from build123d import *

# Parameters (mm, degrees)
SKETCH1_R           = 38.1
SKETCH1_R_2         = 35.1
EXTRUDE_THIN1_DEPTH = 5
BOSS_EXTRUDE1_START = -10
BOSS_EXTRUDE1_DEPTH = 10
SKETCH3_R           = 2.375
CUT_EXTRUDE1_DEPTH  = 10
CIRPATTERN1_COUNT   = 4
SKETCH4_W           = 11
SKETCH4_H           = 10
BOSS_EXTRUDE2_DEPTH = 3
SKETCH5_R           = 2.1
CUT_EXTRUDE2_DEPTH  = 3
CIRPATTERN2_COUNT   = 4
CHAMFER1_SIZE       = 2.178281406
CHAMFER1_SIZE_2     = 2
SKETCH6_R           = 12
BOSS_EXTRUDE3_DEPTH = 5


with BuildPart() as part:
    # Sketch1 → Extrude-Thin1 (new, symmetric)
    with BuildSketch(Plane(origin=(0, 0, 0), x_dir=(1, 0, 0), z_dir=(0, 1, 0))):
        Circle(SKETCH1_R)
        Circle(SKETCH1_R_2, mode=Mode.SUBTRACT)
    extrude(amount=EXTRUDE_THIN1_DEPTH, both=True)

    # Sketch2 → Boss-Extrude1 (add)
    with BuildSketch(Plane(origin=(0, 5, 0), x_dir=(1, 0, 0), z_dir=(0, 1, 0)).offset(BOSS_EXTRUDE1_START)):
        with BuildLine():
            Line((-27.1, 6), (-27.1, -6))
            Line((-27.1, -6), (-33.700938133, -9.811053408))
            ThreePointArc((-33.700938133, -9.811053408), (-35.1, 0), (-33.700938133, 9.811053408))
            Line((-33.700938133, 9.811053408), (-27.1, 6))
        make_face()
    boss_extrude1 = extrude(amount=BOSS_EXTRUDE1_DEPTH)

    # Sketch3 → Cut-Extrude1 (cut)
    with BuildSketch(Plane(origin=(0, 5, 0), x_dir=(1, 0, 0), z_dir=(0, 1, 0))):
        with Locations(Location((-32, 0, 0), (0, 0, 270))):
            Circle(SKETCH3_R)
    cut_extrude1 = extrude(amount=-CUT_EXTRUDE1_DEPTH, mode=Mode.SUBTRACT)

    # CirPattern1: Boss-Extrude1, Cut-Extrude1 ×4 about axis
    cirpattern1_axis = Axis((0, 0, 0), (0, 1, 0))
    add([boss_extrude1.rotate(cirpattern1_axis, i * 360 / CIRPATTERN1_COUNT) for i in range(1, CIRPATTERN1_COUNT)])
    add([cut_extrude1.rotate(cirpattern1_axis, i * 360 / CIRPATTERN1_COUNT) for i in range(1, CIRPATTERN1_COUNT)], mode=Mode.SUBTRACT)

    # Sketch4 → Boss-Extrude2 (add)
    with BuildSketch(Plane.XY):
        with Locations((-42.6, 0)):
            Rectangle(SKETCH4_W, SKETCH4_H)
    boss_extrude2 = extrude(amount=BOSS_EXTRUDE2_DEPTH)

    # Sketch5 → Cut-Extrude2 (cut)
    with BuildSketch(Plane(origin=(0, 0, 0), x_dir=(-1, 0, 0), z_dir=(0, 0, -1))):
        with Locations((43.1, 0)):
            Circle(SKETCH5_R)
    cut_extrude2 = extrude(amount=-CUT_EXTRUDE2_DEPTH, mode=Mode.SUBTRACT)

    # CirPattern2: Boss-Extrude2, Cut-Extrude2 ×4 about axis
    cirpattern2_axis = Axis((0, 0, 0), (0, 1, 0))
    add([boss_extrude2.rotate(cirpattern2_axis, i * 360 / CIRPATTERN2_COUNT) for i in range(1, CIRPATTERN2_COUNT)])
    add([cut_extrude2.rotate(cirpattern2_axis, i * 360 / CIRPATTERN2_COUNT) for i in range(1, CIRPATTERN2_COUNT)], mode=Mode.SUBTRACT)

    # Chamfer1
    # the kernel refuses this chamfer: 2.178281406, 2 mm, written as the material it adds along each edge
    with BuildSketch(Plane(origin=(-3, -5, -37.981706123), x_dir=(-0.9944073694019739, 0, 0.10561242199214178), z_dir=(0, 1, 0))) as chamfer1_piece_1:
        with BuildLine():
            Line((2.056235734, 0), (-CHAMFER1_SIZE * 0.105612421996, -CHAMFER1_SIZE * 0.994407369435))
            Line((-CHAMFER1_SIZE * 0.105612421996, -CHAMFER1_SIZE * 0.994407369435), (0, 0))
            ThreePointArc((0, 0), (1.059779898, -0.013861107), (2.056235734, 0))
        make_face()
    extrude(amount=10)
    with BuildSketch(Plane(origin=(37.981706123, -5, -3), x_dir=(1, 0, 0), z_dir=(0, 1, 0)), Plane(origin=(3, -5, 37.981706123), x_dir=(0, 0, 1), z_dir=(0, 1, 0))) as chamfer1_piece_2:
        with BuildLine():
            Line((CHAMFER1_SIZE, 0), (-0.217164036, 2.044735967))
            ThreePointArc((-0.217164036, 2.044735967), (-0.098142335, 1.055316846), (0, 0))
            Line((0, 0), (CHAMFER1_SIZE, 0))
        make_face()
    extrude(amount=10)
    with BuildSketch(Plane(origin=(-38.1, -5, 0), x_dir=(0.026984720913872013, 0, -0.9996358461145741), z_dir=(0, 1, 0))) as chamfer1_piece_3:
        with BuildLine():
            Line((2.056235734, 0), (-CHAMFER1_SIZE_2 * 0.0269847209139, CHAMFER1_SIZE_2 * 0.999635846115))
            Line((-CHAMFER1_SIZE_2 * 0.0269847209139, CHAMFER1_SIZE_2 * 0.999635846115), (0, 0))
            ThreePointArc((0, 0), (1.057186648, 0.013863174), (2.056235734, 0))
        make_face()
    extrude(amount=10)

    # Sketch6 → Boss-Extrude3 (add, symmetric)
    with BuildSketch(Plane(origin=(0, 0, 0), x_dir=(1, 0, 0), z_dir=(0, 1, 0))):
        with BuildLine():
            Line((-2, 27.1), (-2, 14.866068747))
            ThreePointArc((-2, 14.866068747), (-10.606601718, 10.606601718), (-14.866068747, 2))
            Line((-14.866068747, 2), (-27.1, 2))
            Line((-27.1, 2), (-27.1, -2))
            Line((-27.1, -2), (-14.866068747, -2))
            ThreePointArc((-14.866068747, -2), (-10.606601718, -10.606601718), (-2, -14.866068747))
            Line((-2, -14.866068747), (-2, -27.1))
            Line((-2, -27.1), (2, -27.1))
            Line((2, -27.1), (2, -14.866068747))
            ThreePointArc((2, -14.866068747), (10.606601718, -10.606601718), (14.866068747, -2))
            Line((14.866068747, -2), (27.1, -2))
            Line((27.1, -2), (27.1, 2))
            Line((27.1, 2), (14.866068747, 2))
            ThreePointArc((14.866068747, 2), (10.606601718, 10.606601718), (2, 14.866068747))
            Line((2, 14.866068747), (2, 27.1))
            Line((2, 27.1), (-2, 27.1))
        make_face()
        with Locations(Location((0, 0, 0), (0, 0, 270))):
            Circle(SKETCH6_R, mode=Mode.SUBTRACT)
    extrude(amount=BOSS_EXTRUDE3_DEPTH, both=True)


solid = part.part
Design review of the part built by this model. Coordinates are the model's own, in mm. A direction names the side the tool comes from. Round coordinates to 2 decimals unless told otherwise and drop trailing zeros. Write each loop counter-clockwise with the first axis right and the second up, starting at its lowest first coordinate (ties: lowest second). Pieces come first, ordered by that corner, then holes. Notation, with made-up numbers: (32.25, -30) - (56.25, -30) arc R34 ccw to (56.25, 8) - close; hole circle Ø4 at (76.25, 61). An arc over 180 degrees is marked (long way). Use a Markdown table: item, result. Add a question column.
1. For faces 1 (the face through (-3, 1.2, -45.1)), 2 (the face through (45.4, 0.1, 0)), 3 (the face through (7.932, -0.07, -30.447)), list the 3-axis set-ups (+Z, -Z, +X, -X, +Y, -Y) from which the entire face can be reached by the end or side of a thin tool; tool diameter is ignored.
2. We need section A-A (z = 43.1). State the section outline as (x, y) points.
3. We need section B-B (y = 0). Count the separate pieces of the cut face and the enclosed holes in it, then the cut area to 3 significant figures.
4. We need section C-C (x = 7.5). State the section outline as (y, z) points, then the cut area to 3 significant figures.
5. Mouldability with a two-part tool opening along X and no side actions: class faces 4 (the face through (3, 1.2, 45.1)), 5 (the face through (-39.1, -0.1, -1)), 6 (the face through (27.1, 0, 4)) as +X half, -X half, draft (parallel to the pull), parting line (faces both ways), or undercut.
6. Wall thickness on probe 1 along Z at (x, y) = (-21.5, 3); probe 2 along X at (y, z) = (-3.75, -18): over which ranges is each line inside the solid? List them lowest first.
7. We need section D-D (z = -23.5). State the section outline as (x, y) points.
8. Clearance check with flat-ended pins moving along their axes: pin 1 (10 mm diameter, centred on x = 4, z = -8.5, fed in from +Y); pin 2 (4.5 mm diameter, centred on x = 3, y = -2.5, fed in from -Z); pin 3 (5.5 mm diameter, centred on x = -43.1, y = 0, fed in from -Z); pin 4 (1.2 mm diameter, centred on y = -2.5, z = -4, fed in from +X). State where each tip first meets the part, or that it passes through.
Output:
| question | item | result |
|---|---|---|
| 1 | face 1 | -Z, -X, +Y, -Y |
| 1 | face 2 | +Z, +X, +Y, -Y |
| 1 | face 3 | +Y, -Y |
| 2 | outline | (0, -5) - (3, -5) - (3, -2.1) - (0, -2.1) - close; (0, 2.1) - (3, 2.1) - (3, 5) - (0, 5) - close |
| 3 | separate pieces | 5 |
| 3 | enclosed holes | 9 |
| 3 | area | 1,640 mm2 |
| 4 | outline | (-5, -37.35) - (5, -37.35) - (5, -29.7) - (-5, -29.7) - close; (-5, -12.99) - (5, -12.99) - (5, -9.37) - (-5, -9.37) - close; (-5, 9.37) - (5, 9.37) - (5, 12.99) - (-5, 12.99) - close; (-5, 29.7) - (5, 29.7) - (5, 37.35) - (-5, 37.35) - close |
| 4 | area | 226 mm2 |
| 5 | face 4 | +X half |
| 5 | face 5 | -X half |
| 5 | face 6 | undercut |
| 6 | probe 1 | z = -31.45 to -27.74, -2 to 2, 27.74 to 31.45 |
| 6 | probe 2 | x = -33.58 to -30.13, -2 to 2, 30.13 to 33.58 |
| 7 | outline | (-29.99, -5) - (-26.07, -5) - (-26.07, 5) - (-29.99, 5) - close; (-2, -5) - (2, -5) - (2, 5) - (-2, 5) - close; (26.07, -5) - (29.99, -5) - (29.99, 5) - (26.07, 5) - close |
| 8 | pin 1 | stops at y = 5 |
| 8 | pin 2 | stops at z = -38.09 |
| 8 | pin 3 | stops at z = 0 |
| 8 | pin 4 | stops at x = 39.69 |
